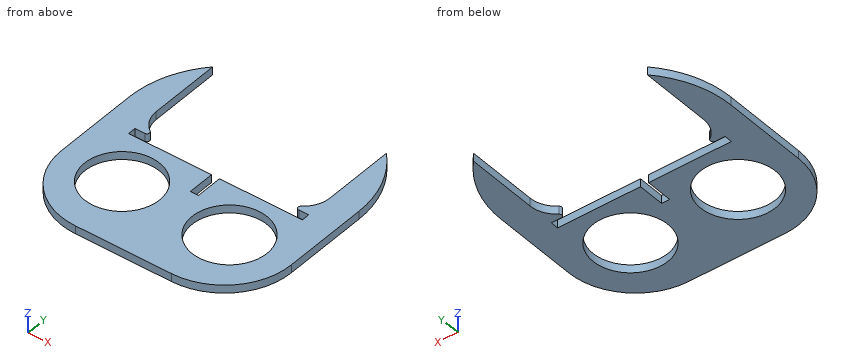
```python
from build123d import *

# Parameters (mm, degrees)
BOSS_EXTRUDE1_DEPTH = 3
CUT_EXTRUDE1_DEPTH  = 10
SKETCH3_W           = 3
SKETCH3_H           = 10
CUT_EXTRUDE2_DEPTH  = 10
SKETCH4_R           = 13.991897225
CUT_EXTRUDE3_DEPTH  = 10
FILLET1_R           = 1


with BuildPart() as part:
    # Sketch1 → Boss-Extrude1 (new body)
    with BuildSketch(Plane.XY):
        with BuildLine():
            Line((-5, 8.5), (5, 8.5))
            ThreePointArc((5, 8.5), (31.870057685, -2.629942315), (43, -29.5))
            Line((43, -29.5), (43, -61.5))
            ThreePointArc((43, -61.5), (35.67766953, -79.17766953), (18, -86.5))
            Line((18, -86.5), (0.5, -86.5))
            Line((0.5, -86.5), (-0.5, -86.5))
            Line((-0.5, -86.5), (-18, -86.5))
            ThreePointArc((-18, -86.5), (-35.67766953, -79.17766953), (-43, -61.5))
            Line((-43, -61.5), (-43, -29.5))
            ThreePointArc((-43, -29.5), (-31.870057685, -2.629942315), (-5, 8.5))
        make_face()
    extrude(amount=BOSS_EXTRUDE1_DEPTH)

    # Sketch2 → Cut-Extrude1 (cut)
    with BuildSketch(Plane.XY.offset(3)):
        with BuildLine():
            Line((-22.5, -40), (22.5, -40))
            ThreePointArc((22.5, -40), (29.571067812, -37.071067812), (32.5, -30))
            Line((32.5, -30), (32.5, 20))
            ThreePointArc((32.5, 20), (29.571067812, 27.071067812), (22.5, 30))
            Line((22.5, 30), (-22.5, 30))
            ThreePointArc((-22.5, 30), (-29.571067812, 27.071067812), (-32.5, 20))
            Line((-32.5, 20), (-32.5, -30))
            ThreePointArc((-32.5, -30), (-29.571067812, -37.071067812), (-22.5, -40))
        make_face()
    extrude(amount=-CUT_EXTRUDE1_DEPTH, mode=Mode.SUBTRACT)

    # Sketch3 → Cut-Extrude2 (cut)
    with BuildSketch(Plane.XY.offset(3)):
        Polygon((-32.5, -40), (-32.5, -43), (-1.5, -43), (1.5, -43), (32.5, -43), (32.5, -40), (22.5, -40), (-22.5, -40), align=None)
        with Locations((0, -48)):
            Rectangle(SKETCH3_W, SKETCH3_H)
    extrude(amount=-CUT_EXTRUDE2_DEPTH, mode=Mode.SUBTRACT)

    # Sketch4 → Cut-Extrude3 (cut)
    with BuildSketch(Plane.XY.offset(3)):
        with Locations((-20.09774362, -61.766309122)):
            Circle(SKETCH4_R)
        with Locations((20.09774362, -61.766309122)):
            Circle(SKETCH4_R)
    extrude(amount=-CUT_EXTRUDE3_DEPTH, mode=Mode.SUBTRACT)

    # Fillet1
    fillet1_edges = [part.edges().sort_by_distance(p)[0] for p in [
        (22.5, -40, 1.5),
        (-22.5, -40, 1.5),
    ]]
    fillet(fillet1_edges, radius=FILLET1_R)


solid = part.part
```
Geometry: final body of the model. Coordinates: model frame, mm. Give positions to 0.01 mm unless a question says otherwise; leave off trailing zeros. Loops run counter-clockwise (first coordinate to the right, second up) from the corner with the lowest first, then second, coordinate; pieces in that order, holes last. Notation, with made-up numbers: (1, 8) -> (50, 8) arc R23 ccw to (50, 43) -> close; hole circle Ø10 at (66, -3.75). An arc over 180 degrees is marked (long way). Use CSV: the item, a comma, the result in double quotes.
(1) Cut plane C-C (y = -58). Output: boundary loops of the cut face in (x, z).
From the geometry:
outline,"(-43, 0) -> (-33.57, 0) -> (-33.57, 3) -> (-43, 3) -> close; (-6.62, 0) -> (6.62, 0) -> (6.62, 3) -> (-6.62, 3) -> close; (33.57, 0) -> (43, 0) -> (43, 3) -> (33.57, 3) -> close"
(2) Cut plane D-D (x = -5). Output: boundary loops of the cut face in (y, z).
From the geometry:
outline,"(-86.5, 0) -> (-43, 0) -> (-43, 3) -> (-86.5, 3) -> close"
(3) Cut plane A-A (y = -10). Output: boundary loops of the cut face in (x, z), plus the area to 3 significant figures.
From the geometry:
outline,"(-37.62, 0) -> (-32.5, 0) -> (-32.5, 3) -> (-37.62, 3) -> close; (32.5, 0) -> (37.62, 0) -> (37.62, 3) -> (32.5, 3) -> close"
area,"30.7 mm^2"
(4) Cut plane B-B (x = 24.5). Output: boundary loops of the cut face in (y, z) (3 decimals).
From the geometry:
outline,"(-85.64, 0) -> (-75.048, 0) -> (-75.048, 3) -> (-85.64, 3) -> close; (-48.485, 0) -> (-43, 0) -> (-43, 3) -> (-48.485, 3) -> close"
(5) First-contact query: P1, Ø8, axis at x = 21.5, y = -39.5, coming from the -Z side; P2, Ø25, axis at x = -20.1, y = -61.77, coming from the +Z side; P3, Ø1.5, axis at x = -15.5, z = 1, coming from the +Y side; P4, Ø0.9, axis at x = 0, z = 2, coming from the +Y side. Flat tips, straight axial feed; report the tip coordinate or a pass-through.
From the geometry:
P1,"z = 0"
P2,"through"
P3,"y = -43"
P4,"y = -53"
(6) Ray query, line 1 along X through (y, z) = (-52.5, 2.2); line 2 along X through (y, z) = (-49.5, 2.65); line 3 along X through (y, z) = (-64.5, 1.6). Return the intervals inside material, ascending. Write a range as [from, to].
From the geometry:
line 1,"[-43, -30.58], [-9.61, -1.5], [1.5, 9.61], [30.58, 43]"
line 2,"[-43, -26.83], [-13.37, -1.5], [1.5, 13.37], [26.83, 43]"
line 3,"[-42.82, -33.82], [-6.38, 6.38], [33.82, 42.82]"
